Job drawing, mm, ordinate dimensions from the low corner. One solid piece. A direction names the side the tool comes from. Coordinates: 2 decimals unless noted, no trailing zeros. Loops run counter-clockwise (first coordinate to the right, second up) from the corner with the lowest first, then second, coordinate; pieces in that order, holes last. Notation, with made-up numbers: (14, 87) -> (63, 87) arc R24 ccw to (63, 113) -> close; hole circle Ø1 at (19.5, 44.5). An arc over 180 degrees is marked (long way). Answer as CSV lines item,"result". Start each with the question number.
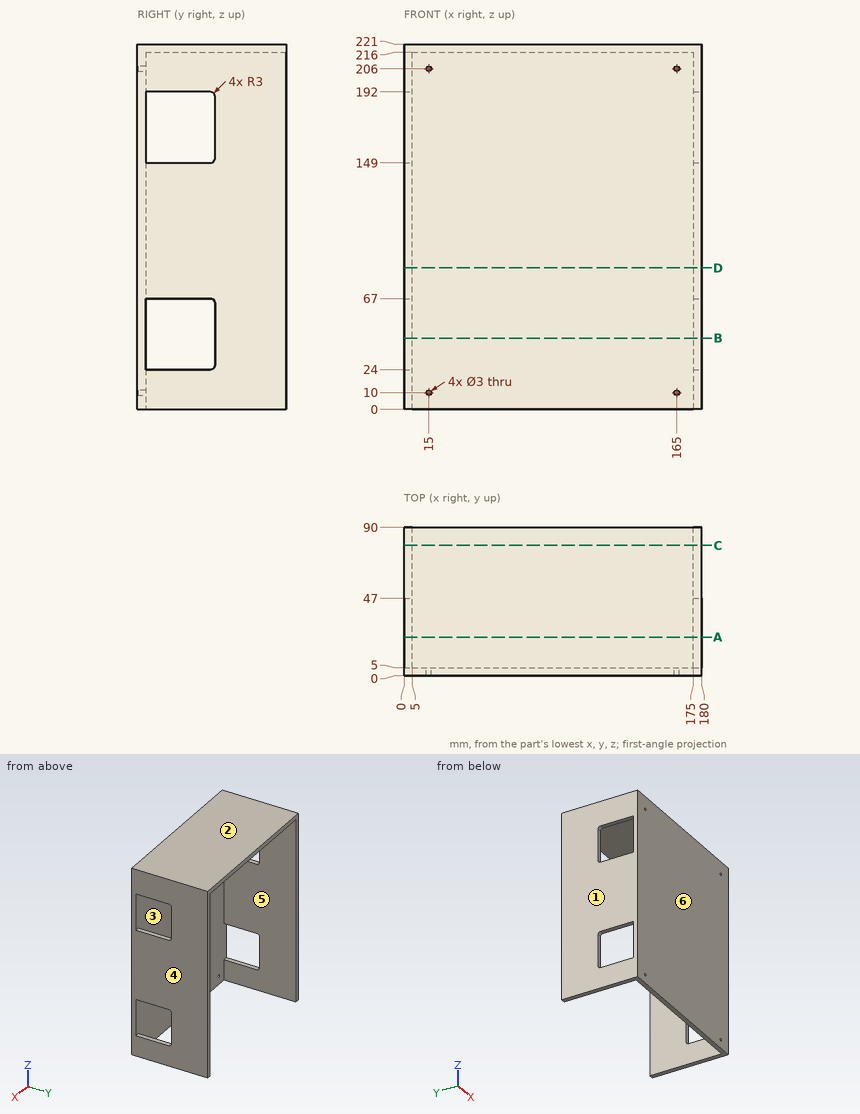
Item 1: Saw through at C-C (y = 79). Write the cut outline in (x, z), plus the area to 3 significant figures.
Item 2: Wall check: probe 1 along X at (y, z) = (2.65, 10); probe 2 along Z at (x, y) = (165, 2.7); probe 3 along X at (y, z) = (51.5, 152). Give the ranges that are in metal, low to high.
Item 3: Saw through at D-D (z = 85.5). Write the cut outline in (x, y).
Item 4: Saw through at A-A (y = 23.5). Write the cut outline in (x, z), plus the area to 3 significant figures.
Item 5: Which spindle directions (+Z, -Z, +X, -X, +Y, -Y) get a long thin tool onto all of the face, cutting with end or side? Do the marked faces 5 and 6. Say none if no direction does.
Item 6: Saw through at B-B (z = 43). Write the cut outline in (x, y), plus the area to 3 significant figures.
Item 7: Flat gauge pins, fed straight in: pin 1 Ø2.5 at (x, z) = (15, 206) entering from -Y; pin 2 Ø8 at (x, z) = (122.5, 136.5) entering from +Y; pin 3 Ø8 at (x, z) = (52, 112) entering from -Y. Where does each tip first touch, or does it go through?
Item 8: Two-plate mould, pull along X, no slides. Class the marked faces 1, 2, 3 and 4: pulls with the +X half, pulls with the -X half, needs draft (parallel to the pull), parting line crosses it, or undercut.
Geometry check:
1,outline,"(0, 0) -> (5, 0) -> (5, 216) -> (175, 216) -> (175, 0) -> (180, 0) -> (180, 221) -> (0, 221) -> close"
1,area,"3,060 mm2"
2,probe 1,"0 to 13.5, 16.5 to 163.5, 166.5 to 180"
2,probe 2,"0 to 8.5, 11.5 to 204.5, 207.5 to 221"
2,probe 3,"0 to 5, 175 to 180"
3,outline,"(0, 0) -> (180, 0) -> (180, 90) -> (175, 90) -> (175, 5) -> (5, 5) -> (5, 90) -> (0, 90) -> close"
4,outline,"(0, 0) -> (5, 0) -> (5, 24) -> (0, 24) -> close; (0, 67) -> (5, 67) -> (5, 149) -> (0, 149) -> close; (0, 192) -> (5, 192) -> (5, 216) -> (175, 216) -> (175, 192) -> (180, 192) -> (180, 221) -> (0, 221) -> close; (175, 0) -> (180, 0) -> (180, 24) -> (175, 24) -> close; (175, 67) -> (180, 67) -> (180, 149) -> (175, 149) -> close"
4,area,"2,200 mm2"
5,face 5,"-Z, +Y"
5,face 6,"+Z, -Z, +X, -X, -Y"
6,outline,"(0, 0) -> (180, 0) -> (180, 5) -> (0, 5) -> close; (0, 47) -> (5, 47) -> (5, 90) -> (0, 90) -> close; (175, 47) -> (180, 47) -> (180, 90) -> (175, 90) -> close"
6,area,"1,330 mm2"
7,pin 1,"through"
7,pin 2,"y = 5"
7,pin 3,"y = 0"
8,face 1,"pulls with the -X half"
8,face 2,"needs draft"
8,face 3,"undercut"
8,face 4,"pulls with the +X half"
